Check sheet for the modelled part. Datum: model origin and axes. Units: mm. Face numbers are marked on the shaded views. A direction names the side the tool comes from. Coordinates: 2 decimals unless noted, no trailing zeros. Write each loop counter-clockwise with the first axis right and the second up, starting at its lowest first coordinate (ties: lowest second). Pieces come first, ordered by that corner, then holes. Notation, with made-up numbers: (40.5, 24.25) -> (98.5, 24.25) arc R18 cw to (98.5, 34.25) -> close; hole circle Ø2 at (-30.5, 39.25). An arc over 180 degrees is marked (long way). Put each result on its own line as item: value.
```python
from build123d import *

# Parameters (mm, degrees)
F1_DEPTH = 25.4
F2_W     = 6.35
F2_H     = 12.7
F3_DEPTH = 6.351
F4_W     = 19.05
F4_H     = 12.7
F5_DEPTH = 12.701


with BuildPart() as f1:
    # F0 (on Front) → F1 (new body)
    with BuildSketch(Plane.XZ):
        Polygon((0, 25.4), (0, 0), (50.8, 0), (50.8, 12.7), (6.35, 12.7), (6.35, 25.4), align=None)
    extrude(amount=F1_DEPTH)

    # F2 (on face) → F3 (cut, through all)
    with BuildSketch(Plane.YZ.offset(6.35)):
        with Locations((-22.225, 19.05)):
            Rectangle(F2_W, F2_H)
    extrude(amount=-F3_DEPTH, mode=Mode.SUBTRACT)

    # F4 (on face) → F5 (cut, through all)
    with BuildSketch(Plane.XY.offset(12.7)):
        with Locations((41.275, -19.05)):
            Rectangle(F4_W, F4_H)
    extrude(amount=-F5_DEPTH, mode=Mode.SUBTRACT)


solid = f1.part
```
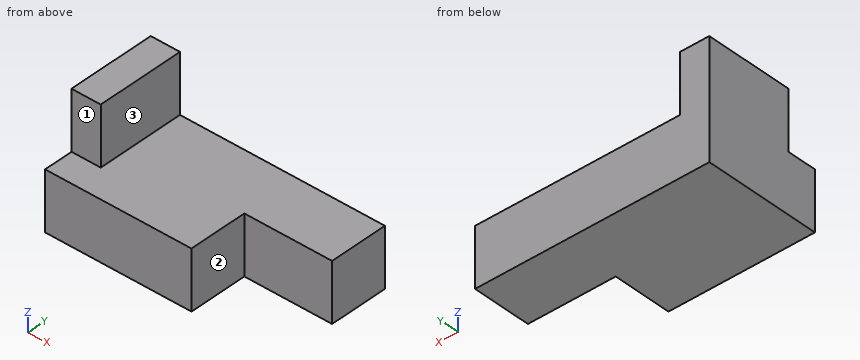
Q1. Cross-section at B-B (z = 12). Record the cut outline in (x, y), plus the area to 3 significant figures.
Recorded:
outline: (0, -25.4) -> (31.75, -25.4) -> (31.75, -12.7) -> (50.8, -12.7) -> (50.8, 0) -> (0, 0) -> close
area: 1,050 mm2
Q2. Cross-section at D-D (y = -22.5). Record the cut outline in (x, z), plus the area to 3 significant figures.
Recorded:
outline: (0, 0) -> (31.75, 0) -> (31.75, 12.7) -> (0, 12.7) -> close
area: 403 mm2
Q3. Depth check by flat-ended pin: P1, Ø8, axis at y = -11, z = 14.5, coming from the -X side; P2, Ø10, axis at x = 34.5, y = -21.5, coming from the +Z side; P3, Ø6.5, axis at y = -19, z = 9.5, coming from the +X side; P4, Ø10, axis at x = 45, z = 19.5, coming from the +Y side. Enter the tip coordinate at first touch or a pass-through.
Recorded:
P1: stops at x = 0
P2: stops at z = 12.7
P3: stops at x = 31.75
P4: passes through
Q4. Cross-section at C-C (x = 41). Record the cut outline in (y, z).
Recorded:
outline: (-12.7, 0) -> (0, 0) -> (0, 12.7) -> (-12.7, 12.7) -> close
Q5. Cross-section at A-A (y = -16.5). Record the cut outline in (x, z).
Recorded:
outline: (0, 0) -> (31.75, 0) -> (31.75, 12.7) -> (6.35, 12.7) -> (6.35, 25.4) -> (0, 25.4) -> close
Q6. Material ranges on line 1 along X through (y, z) = (-1.75, 18); line 2 along Y through (x, z) = (41, 10.25); line 3 along Z through (x, y) = (33, -6.5), recorded low to high.
Recorded:
line 1: x = 0 to 6.35
line 2: y = -12.7 to 0
line 3: z = 0 to 12.7
Q7. Tool access check on the marked faces 1, 2 and 3. Record the directions out of +Z, -Z, +X, -X, +Y, -Y that give a thin tool (end or side, any length) a straight path to the whole face; none if there is none.
Recorded:
face 1: +Z, +X, -X, -Y
face 2: +Z, -Z, +X, -Y
face 3: +Z, +X, +Y, -Y
